```python
from build123d import *

# Parameters (mm, degrees)
F0_W     = 10
F0_H     = 10
F1_DEPTH = 20
F2_W     = 10
F2_H     = 10
F3_DEPTH = 495
F4_W     = 350
F4_H     = 4
F5_DEPTH = 30
F7_DEPTH = 7.001
F9_DEPTH = 7.001


with BuildPart() as f1:
    # F0 (on Top) → F1 (new body)
    with BuildSketch(Plane.XY):
        Rectangle(F0_W, F0_H)
    extrude(amount=-F1_DEPTH)

    # F2 (on face) → F3 (join)
    with BuildSketch(Plane(origin=(-5, 0, 0), x_dir=(0, -1, 0), z_dir=(-1, 0, 0))):
        with Locations((0, -15)):
            Rectangle(F2_W, F2_H)
    extrude(amount=F3_DEPTH)

    # F4 (on face) → F5 (join)
    with BuildSketch(Plane(origin=(0, 0, -20), x_dir=(1, 0, 0), z_dir=(0, 0, -1))):
        with Locations((-325, 0)):
            Rectangle(F4_W, F4_H)
    extrude(amount=F5_DEPTH)

    # F6 (on face) → F7 (cut, through all)
    with BuildSketch(Plane.XZ.offset(2)):
        Polygon((-150, -50), (-150, -20), (-500, -50), align=None)
    extrude(amount=-F7_DEPTH, mode=Mode.SUBTRACT)

    # F8 (on face) → F9 (cut, through all)
    with BuildSketch(Plane.XZ.offset(2)):
        Polygon((-500, -20), (-500, -40), (-266.666667, -20), align=None)
    extrude(amount=-F9_DEPTH, mode=Mode.SUBTRACT)


solid = f1.part
```
Model file for the job. Use its own axes, mm. A direction names the side the tool comes from. Coordinates: 2 decimals unless noted, no trailing zeros. Order: outer loops, then holes, each group sorted by start corner. A loop starts at its lowest first (then second) coordinate and runs counter-clockwise, first axis right, second up. Notation, with made-up numbers: (60, 5) -> (93, 5) arc R17 cw to (93, 31) -> close; hole circle Ø6 at (0.5, 20). An arc over 180 degrees is marked (long way). Answer as a JSON object with one key per item and string values. Group by question number.
1) Cut at C-C, the plane x = -195.5. Write the cut outline in (y, z), then the cut area to 3 significant figures.
2) Drill centre lines: L1, parallel to Z at x = -108, y = -1.75; L2, parallel to X at y = 2.5, z = -8.5; L3, parallel to Y at x = -423, z = -41. Where is each one in solid material? Low to high.
3) Cut at B-B, the plane y = -0.5. Write the cut outline in (x, z), then the cut area to 3 significant figures.
4) Flat gauge pins, fed straight in: pin 1 (1 mm diameter, centred on y = 3, z = -32.5, fed in from +X); pin 2 (15 mm diameter, centred on x = -327.5, z = -29, fed in from -Y); pin 3 (3 mm diameter, centred on y = -0.5, z = -5.5, fed in from -X); pin 4 (5 mm diameter, centred on x = -157, y = -0.5, fed in from -Z). Where does each tip first touch, or does it go through?
5) Which spindle directions (+Z, -Z, +X, -X, +Y, -Y) get a long thin tool onto all of the face, cutting with end or side? Do faces 5 (the face through (5, 0, -10)), 6 (the face through (-352, -2, -32)), 7 (the face through (-249, 0, -10)). Say none if no direction does.
6) Cut at A-A, the plane x = -437.5. Write the cut outline in (y, z).
7) Pull direction Z, two halves, no side cores. Call faces 1 (the face through (-244, 2.3, -20)), 2 (the face through (-384.97, -0.03, -30.14)), 3 (the face through (-322.55, -0.03, -34.79)), 4 (the face through (-352, 2, -32)): +Z half, -Z half, draft (parallel to the pull), parting line (faces both ways), or undercut.
8) Cut at D-D, the plane z = -4.5. Write the cut outline in (x, y), then the cut area to 3 significant figures.
Check values:
{
 "1": {"outline": "(-5, -20) -> (-2, -20) -> (-2, -23.9) -> (2, -23.9) -> (2, -20) -> (5, -20) -> (5, -10) -> (-5, -10) -> close", "area": "116 mm²"},
 "2": {"L1": "z = -20 to -10", "L2": "x = -5 to 5", "L3": "y = -2 to 2"},
 "3": {"outline": "(-500, -50) -> (-150, -20) -> (5, -20) -> (5, 0) -> (-5, 0) -> (-5, -10) -> (-500, -10) -> (-500, -20) -> (-266.67, -20) -> (-500, -40) -> close", "area": "8,070 mm²"},
 "4": {"pin 1": "passes through", "pin 2": "stops at y = -2", "pin 3": "stops at x = -5", "pin 4": "stops at z = -20.81"},
 "5": {"face 5": "+Z, -Z, +X, +Y, -Y", "face 6": "-Z, +X, -X, -Y", "face 7": "+Z, -X, +Y, -Y"},
 "6": {"outline": "(-5, -20) -> (5, -20) -> (5, -10) -> (-5, -10) -> close; (-2, -44.64) -> (2, -44.64) -> (2, -34.64) -> (-2, -34.64) -> close"},
 "7": {"face 1": "undercut", "face 2": "undercut", "face 3": "-Z half", "face 4": "draft"},
 "8": {"outline": "(-5, -5) -> (5, -5) -> (5, 5) -> (-5, 5) -> close", "area": "100 mm²"}
}
